Design review of the part built by this model. Coordinates are the model's own, in mm. Coordinates: 2 decimals unless noted, no trailing zeros. Loops run counter-clockwise (first coordinate to the right, second up) from the corner with the lowest first, then second, coordinate; pieces in that order, holes last. Notation, with made-up numbers: M 45,2.25 L 58,2.25 A36 ccw 58,38.25 Z; hole C -24,-25.75 d10. An arc over 180 degrees is marked long. Write item = value, one per line. Start each with the question number.
Autodesk Inventor part; units mm, degrees
ref_plane "YZ Plane" through (0, 0, 0) normal (1, 0, 0) x (0, 1, 0)
ref_plane "XZ Plane" through (0, 0, 0) normal (0, 1, 0) x (-1, 0, 0)
ref_plane "XY Plane" through (0, 0, 0) normal (0, 0, 1) x (1, 0, 0)
sketch "Эскиз1" plane through (0, 0, 0) normal (0, 0, 1) x (1, 0, 0)
  circle A0 centre (0, 0) radius 6
  circle A1 centre (18, 0) radius 7.5
  line L0 (0, 0) -> (18, 0)
  line L1 (0, 0) -> (18, 0) construction
  line L2 (-0.5, -8.9861) -> (17.4444, -9.9846)
  line L3 (17.4444, 9.9846) -> (-0.5, 8.9861)
  arc A2 (-0.5, 8.9861) -> (-0.5, -8.9861) centre (0, 0) ccw
  arc A3 (17.4444, -9.9846) -> (17.4444, 9.9846) centre (18, 0) ccw
  point P0 (9, 0)
  dimension "d0" = 12
  dimension "d1" = 15
  dimension "d2" = 18
  dimension "d4" = 9
  dimension "d7" = 10
extrude "Выдавливание1" add sketch "Эскиз1" along normal blind 6
properties part number "Крепление линейного подшипника"
(1) Take a section at A-A (y = 0). State the section outline as (x, z) points, plus the area to 3 significant figures.
(2) Take a section at C-C (z = 1.8). State the section outline as (x, y) points, plus the area to 3 significant figures.
(3) Take a section at D-D (x = -4.5). State the section outline as (y, z) points, plus the area to 3 significant figures.
(4) Mouldability with a two-part tool opening along Y and no side actions: class faces 1 (the flat face through (8.598, 9.492, 2.958)), 2 (the cylindrical face through (-6, 0, 3)), 3 (the flat face through (9, 0, 0)) as +Y half, -Y half, draft (parallel to the pull), parting line (faces both ways), or undercut.
(5) To check wall thickness, follow L1, parallel to Y at x = 18, z = 4.1; L2, parallel to X at y = 1, z = 1.4; L3, parallel to X at y = 3.5, z = 2.7. State the ranges of each line that lie inside material, in increasing order.
(6) Take a section at B-B (x = 18). State the section outline as (y, z) points, plus the area to 3 significant figures.
(7) Insertion check: pin 1 (3 mm diameter, centred on y = -6.5, z = 4, fed in from +X); pin 2 (1.5 mm diameter, centred on y = -4, z = 1, fed in from +X). Each pin has a flat end and moves straight along its axis. Give the tip position at first contact, or say it passes through.
Results list:
q1.outline = M -9,0 L -6,0 L -6,6 L -9,6 Z; M 6,0 L 10.5,0 L 10.5,6 L 6,6 Z; M 25.5,0 L 28,0 L 28,6 L 25.5,6 Z
q1.area = 60.0 mm^2
q2.outline = M -0.5,-8.99 L 17.44,-9.98 A10 ccw long 17.44,9.98 L -0.5,8.99 A9 ccw Z; hole C 0,0 d12; hole C 18,0 d15
q2.area = 337 mm^2
q3.outline = M -7.79,0 L -3.97,0 L -3.97,6 L -7.79,6 Z; M 3.97,0 L 7.79,0 L 7.79,6 L 3.97,6 Z
q3.area = 45.9 mm^2
q4.face_1 = +Y half
q4.face_2 = undercut
q4.face_3 = draft
q5.L1 = -10 to -7.5, 7.5 to 10
q5.L2 = -8.94 to -5.92, 5.92 to 10.57, 25.43 to 27.95
q5.L3 = -8.29 to -4.87, 4.87 to 11.37, 24.63 to 27.37
q6.outline = M -10,0 L -7.5,0 L -7.5,6 L -10,6 Z; M 7.5,0 L 10,0 L 10,6 L 7.5,6 Z
q6.area = 30.0 mm^2
q7.pin_1 = 26.66
q7.pin_2 = 27.46
